Geometry: final body of the model. Coordinates: model frame, mm. A direction names the side the tool comes from. Give positions to 0.01 mm unless a question says otherwise; leave off trailing zeros. Write each loop counter-clockwise with the first axis right and the second up, starting at its lowest first coordinate (ties: lowest second). Pieces come first, ordered by that corner, then holes. Notation, with made-up numbers: M 70,-26 L 80,-26 A19 ccw 80,-1 Z; hole C 30,39 d2. An arc over 180 degrees is marked long. Use one line per item in the form item = value. Start each with the question number.
Item 1: Section query C-C on y = 0. Return loops of the section in (x, z) (3 decimals).
Item 2: Access query for faces 4 (the flat face through (35, -50, 0)), 5 (the flat face through (-35, 50, 0)), 6 (the flat face through (-24.6, -50.3, 24.9)). Directions: +Z, -Z, +X, -X, +Y, -Y. A direction counts if a zero-diameter tool reaches every point of the face in a straight line with its end or side. Return the directions, or none.
Item 3: Contact query for flat-ended pins moving along their axis: P1, Ø2, axis at y = -4.5, z = 7.5, coming from the -X side; P2, Ø1, axis at x = 9.5, z = 52.5, coming from the -Y side; P3, Ø1.5, axis at y = 2.5, z = 104, coming from the +X side; P4, Ø23, axis at x = -0.5, y = -58.5, coming from the +Z side (3 decimals). Output: stop coordinate, or through.
Item 4: Section query D-D on y = -26. Give the number of separate pieces and of enclosed holes in the cut face, then the cut area to 3 significant figures.
Item 5: Material intervals for line 1 along Z through (x, y) = (0, -34); line 2 along Z through (x, y) = (0, -65); line 3 along X through (y, z) = (-65, 0), sorted ascending. Write a range as from..to.
Item 6: Pull-direction query (Y, two-part tool) for faces 1 (the flat face through (-1, -1, 198)), 2 (the flat face through (0, -50, -35)), 3 (the flat face through (24, -70, 16)); classes: released by +Y, released by -Y, zero draft, split by the parting line, or undercut.
Item 7: Section query B-B on z = 0. Return loops of the section in (x, y).
Autodesk Inventor part; units mm, degrees
ref_plane "YZ Plane" through (0, 0, 0) normal (1, 0, 0) x (0, 1, 0)
ref_plane "XZ Plane" through (0, 0, 0) normal (0, 1, 0) x (-1, 0, 0)
ref_plane "XY Plane" through (0, 0, 0) normal (0, 0, 1) x (1, 0, 0)
sketch "Sketch3" plane through (0, 0, 0) normal (0, 1, 0) x (-1, 0, 0)
  line L0 (-14.4975, 35) -> (14.4975, 35)
  line L1 (14.4975, 35) -> (35, 14.4975)
  line L2 (35, 14.4975) -> (35, -14.4975)
  line L3 (35, -14.4975) -> (14.4975, -35)
  line L4 (14.4975, -35) -> (-14.4975, -35)
  line L5 (-14.4975, -35) -> (-35, -14.4975)
  line L6 (-35, -14.4975) -> (-35, 14.4975)
  line L7 (-35, 14.4975) -> (-14.4975, 35)
  circle A0 centre (0, 0) radius 37.8837
  circle A1 centre (0, 0) radius 35
  circle A2 centre (0, 0) radius 26
  circle A3 centre (0, 0) radius 39.8837
  line L8 (0, 0) -> (-35, 0)
  line L9 (-35, 0) -> (-35, 96.5)
  line L10 (-35, 96.5) -> (0, 96.5)
  line L11 (0, 96.5) -> (0, 0)
  line L12 (0, 96.5) -> (-9.665, 96.5)
  line L13 (-9.665, 96.5) -> (-9.665, 193)
  line L14 (-9.665, 193) -> (0, 193)
  line L15 (0, 193) -> (0, 96.5)
  line L16 (0, 193) -> (-60, 193)
  line L17 (-60, 193) -> (-60, 198)
  line L18 (-60, 198) -> (0, 198)
  line L19 (0, 198) -> (0, 193)
  circle A4 centre (-60, 195.5) radius 9.665
  dimension "oSW" = 70
  dimension "oIntDia" = 52
  dimension "d16" = 2
  dimension "oWheelDia" = 120
  dimension "d51" = 5
  dimension "d52" = 19.33
  dimension "oStemHeight" = 198
  dimension "d57" = 19.33
  dimension "d58" = 28.9949
revolve "Revolution1" add sketch "Sketch3" angle 360 about axis through (0, 0, 193) along (0, 0, -1) picked at (-8.1008, 35.5309) picked at (-33.833, 18.2227) picked at (-2.2761, 31.7758) picked at (-17.116, 1.9285) contours A0 L11 L0 | L0 A1 L7 | L7 A0 | A0 L9 A3 L11 | L11 A2 L8 A1 | A1 L6 L7 | L11 L8 A2 | L9 L10 L11 A3 | L10 L13 L14 L15 | L14 L16 A4 L18 L19 | A4 L18 L17 L16 | L16 L17 L18 A4
extrude "Extrusion1" add sketch "Sketch3" along normal mid plane 140 separate body contours L0 A1 L7 | L0 L1 A1 | L11 A2 L8 A1 | A1 L8 A2 L11 | A1 L6 L7 | L1 L2 A1 | A1 L5 L6 | L2 L3 A1 | A1 L4 L5 | L3 L4 A1
extrude "Extrusion12" cut sketch "Sketch3" along normal through all both and the other way through all contours L11 L8 A2 | A2 L8 L11
extrude "Extrusion2" add sketch "Sketch3" along normal mid plane 60 contours A0 L11 L0 | L7 A0 | A0 L9 A3 L11 | L11 A0 L0 | L6 A0 | A0 L11 A3 L9 | A0 L1 | L5 A0 | A0 L2 | L4 A0 | A0 L3
sketch "Sketch10" plane through (0, 70, 0) normal (0, 1, 0) x (1, 0, 0)
  circle A0 centre (0, 0) radius 26
  circle A1 centre (0, 0) radius 26.25
  dimension "d44" = 0.25
extrude "Extrusion11" cut sketch "Sketch10" against normal blind 12
mirror "Mirror1" about plane through (0, 0, 0) normal (0, 1, 0) of "Extrusion11"
equation "\"d52\" = 0.666667 * d58"
equation "\"d57\" = d52"
properties part number "Manual Threaded Globe Valve DN50 S235" material "S235"
Answer sheet:
q1.outline = M -50.664,193 L -9.665,193 L -9.665,96.5 L -35,96.5 L -35,19.124 A39.884 ccw long 35,19.124 L 35,96.5 L 9.665,96.5 L 9.665,193 L 50.664,193 A9.665 ccw long 50.664,198 L -50.664,198 A9.665 ccw long Z; hole C 0,0 d52
q2.face_4 = -Z, +X, -Y
q2.face_5 = -Z, -X, +Y
q2.face_6 = -X, -Y
q3.P1 = -39.35
q3.P2 = -33.82
q3.P3 = 9.51
q3.P4 = 205.165
q4.separate_pieces = 2
q4.enclosed_holes = 1
q4.area = 6,730 mm2
q5.line_1 = -35..-26, 26..96.5, 193..198
q5.line_2 = -35..-26.25, 26.25..35, 187.23..203.77
q5.line_3 = -35..-26.25, 26.25..35
q6.face_1 = undercut
q6.face_2 = zero draft
q6.face_3 = released by -Y
q7.outline = M -39.88,-30 L -35,-30 L -35,-70 L -26.25,-70 L -26.25,-58 L -26,-58 L -26,58 L -26.25,58 L -26.25,70 L -35,70 L -35,30 L -39.88,30 Z; M 26,-58 L 26.25,-58 L 26.25,-70 L 35,-70 L 35,-30 L 39.88,-30 L 39.88,30 L 35,30 L 35,70 L 26.25,70 L 26.25,58 L 26,58 Z
